Can you work these out from the model? Positions are in its coordinate system, mm. A direction names the side the tool comes from. Give positions to 0.01 mm unless a question says otherwise; leave off trailing zeros. Order: outer loops, then holes, each group sorted by start corner. A loop starts at its lowest first (then second) coordinate and runs counter-clockwise, first axis right, second up.
Item 1: If we mould it in two halves opening along Y, with no side actions, what happens to faces 1 (the flat face through (-20, 1, 2)), 2 (the cylindrical face through (-0.238, -31.074, 1.521)), 3 (the flat face through (14, -10, 2)), 4 (the cylindrical face through (-0.238, -16.074, 1.521))? For each: +Y half, -Y half, draft (parallel to the pull), parting line (faces both ways), or undercut.
Item 2: I want a section at B-B, the plane y = -15. Write out the boundary of the cut face in (x, z).
Item 3: I'm going to push flat-ended pins straight in: pin 1 Ø1.5 at (y, z) = (26.5, 1) entering from +X; pin 2 Ø1.5 at (y, z) = (38.5, 2) entering from -X; pin 3 Ø1.5 at (y, z) = (-13, 1) entering from +X. Where does each tip first touch, or does it pass through?
Item 4: Which directions (+Z, -Z, +X, -X, +Y, -Y) give clear straight access to the entire face, cutting with the end or side of a thin tool? Please do faces 5 (the flat face through (-8, -30, 2)), 6 (the cylindrical face through (-8.9, 12.86, 1.48)), 7 (the flat face through (8, 31, 2)).
Item 5: If I drill on line 1 along X through (y, z) = (22.5, 0.2); line 2 along Y through (x, z) = (15, 1.5); line 3 along Y through (x, z) = (-12, 2.8), over which ranges is the centre line in solid material (lowest first)?
Item 6: I want a section at C-C, the plane z = 2. Count the separate pieces of the cut face and the enclosed holes in it, then the cut area to 3 significant figures.
Item 7: I want a section at A-A, the plane x = -15. Write out the boundary of the cut face in (y, z).
```python
from build123d import *

# Parameters (mm, degrees)
SKETCH_1_W          = 40
SKETCH_1_H          = 150
SKETCH_1_R          = 1.6
EXTRUDE_1_DEPTH     = 3
SKETCH_2_R          = 1.1
CUT_EXTRUDE_1_DEPTH = 4
SKETCH_4_W          = 40
SKETCH_4_H          = 18
CUT_EXTRUDE_3_DEPTH = 10
SKETCH_5_W          = 40
SKETCH_5_H          = 12
EXTRUDE_2_DEPTH     = 3
SKETCH_6_R          = 1.1
CUT_EXTRUDE_4_DEPTH = 10
SKETCH_7_W          = 12
SKETCH_7_H          = 75
SKETCH_7_H_2        = 47
CUT_EXTRUDE_5_DEPTH = 10
FILLET_1_R          = 3
SKETCH_8_W          = 16
SKETCH_8_H          = 42.139164074
SKETCH_8_H_2        = 21.417935282
CUT_EXTRUDE_6_DEPTH = 10
FILLET_2_R          = 4


with BuildPart() as part:
    # 草图1 → 凸台-拉伸1 (new body)
    with BuildSketch(Plane.XY):
        Rectangle(SKETCH_1_W, SKETCH_1_H)
        with Locations((-15, 0)):
            Circle(SKETCH_1_R, mode=Mode.SUBTRACT)
        with Locations((15, 0)):
            Circle(SKETCH_1_R, mode=Mode.SUBTRACT)
    extrude(amount=EXTRUDE_1_DEPTH)

    # 草图2 → 切除-拉伸1 (cut, through all)
    with BuildSketch(Plane.XY.offset(3)):
        with Locations((0, 30)):
            Circle(SKETCH_2_R)
        with Locations((0, 45)):
            Circle(SKETCH_2_R)
        with Locations((0, 60)):
            Circle(SKETCH_2_R)
        with Locations((0, 15)):
            Circle(SKETCH_2_R)
        with Locations((0, -15)):
            Circle(SKETCH_2_R)
        Circle(SKETCH_2_R)
        with Locations((0, -30)):
            Circle(SKETCH_2_R)
        with Locations((0, -45)):
            Circle(SKETCH_2_R)
        with Locations((0, -60)):
            Circle(SKETCH_2_R)
    extrude(amount=-CUT_EXTRUDE_1_DEPTH, mode=Mode.SUBTRACT)

    # 草图4 → 切除-拉伸3 (cut)
    with BuildSketch(Plane.XY.offset(3)):
        with Locations((0, -66)):
            Rectangle(SKETCH_4_W, SKETCH_4_H)
    extrude(amount=-CUT_EXTRUDE_3_DEPTH, mode=Mode.SUBTRACT)

    # 草图5 → 凸台-拉伸2 (add)
    with BuildSketch(Plane.XY.offset(3)):
        with Locations((0, 81)):
            Rectangle(SKETCH_5_W, SKETCH_5_H)
    extrude(amount=-EXTRUDE_2_DEPTH)

    # 草图6 → 切除-拉伸4 (cut)
    with BuildSketch(Plane.XY.offset(3)):
        with Locations((0, 75)):
            Circle(SKETCH_6_R)
    extrude(amount=-CUT_EXTRUDE_4_DEPTH, mode=Mode.SUBTRACT)

    # 草图7 → 切除-拉伸5 (cut)
    with BuildSketch(Plane.XY.offset(3)):
        with Locations((-14, 49.5)):
            Rectangle(SKETCH_7_W, SKETCH_7_H)
        with Locations((-14, -33.5)):
            Rectangle(SKETCH_7_W, SKETCH_7_H_2)
        with Locations((14, -33.5)):
            Rectangle(SKETCH_7_W, SKETCH_7_H_2)
        with Locations((14, 49.5)):
            Rectangle(SKETCH_7_W, SKETCH_7_H)
    extrude(amount=-CUT_EXTRUDE_5_DEPTH, mode=Mode.SUBTRACT)

    # 圆角1
    fillet_1_edges = [part.edges().sort_by_distance(p)[0] for p in [
        (-8, 87, 1.5),
        (8, 87, 1.5),
        (-8, -57, 1.5),
        (8, -57, 1.5),
        (20, 12, 1.5),
        (8, 12, 1.5),
        (8, -10, 1.5),
        (20, -10, 1.5),
        (-20, -10, 1.5),
        (-8, -10, 1.5),
        (-20, 12, 1.5),
        (-8, 12, 1.5),
    ]]
    fillet(fillet_1_edges, radius=FILLET_1_R)

    # 草图8 → 切除-拉伸6 (cut)
    with BuildSketch(Plane.XY.offset(3)):
        with Locations((0, 73.069582037)):
            Rectangle(SKETCH_8_W, SKETCH_8_H)
        with Locations((0, -60.708967641)):
            Rectangle(SKETCH_8_W, SKETCH_8_H_2)
    extrude(amount=-CUT_EXTRUDE_6_DEPTH, mode=Mode.SUBTRACT)

    # 圆角2
    fillet_2_edges = [part.edges().sort_by_distance(p)[0] for p in [
        (8, 52, 1.5),
        (-8, 52, 1.5),
        (8, -50, 1.5),
        (-8, -50, 1.5),
    ]]
    fillet(fillet_2_edges, radius=FILLET_2_R)


solid = part.part
```
Results list:
1. face 1: draft
1. face 2: undercut
1. face 3: -Y half
1. face 4: undercut
2. outline: (-8, 0) - (-1.1, 0) - (-1.1, 3) - (-8, 3) - close; (1.1, 0) - (8, 0) - (8, 3) - (1.1, 3) - close
3. pin 1: stops at x = 8
3. pin 2: stops at x = -8
3. pin 3: stops at x = 8.1
4. face 5: +Z, -Z, -X, -Y
4. face 6: +Z, -Z, -X, +Y
4. face 7: +Z, -Z, +X, +Y
5. line 1: x = -8 to 8
5. line 2: y = -10 to -1.6, 1.6 to 12
5. line 3: y = -10 to 12
6. separate pieces: 1
6. enclosed holes: 9
6. area: 2,100 mm2
7. outline: (-10, 0) - (-1.6, 0) - (-1.6, 3) - (-10, 3) - close; (1.6, 0) - (12, 0) - (12, 3) - (1.6, 3) - close
